from build123d import *

# Parameters (mm, degrees)
F0_W     = 88.9
F0_H     = 38.1
F1_DEPTH = 222.25
F2_R     = 9.525
F3_DEPTH = 12.7
F4_R     = 9.525
F5_DEPTH = 12.7


with BuildPart() as f1:
    # F0 (on Front) → F1 (new body, symmetric)
    with BuildSketch(Plane.XZ):
        Rectangle(F0_W, F0_H)
    extrude(amount=F1_DEPTH, both=True)

    # F2 (on face) → F3 (cut)
    with BuildSketch(Plane.XY.offset(19.05)):
        with Locations((0, 177.8)):
            Circle(F2_R)
        with Locations((0, -177.8)):
            Circle(F2_R)
    extrude(amount=-F3_DEPTH, mode=Mode.SUBTRACT)

    # F4 (on face) → F5 (cut)
    with BuildSketch(Plane(origin=(0, 0, -19.05), x_dir=(1, 0, 0), z_dir=(0, 0, -1))):
        with Locations((0, -177.8)):
            Circle(F4_R)
        with Locations((0, 177.8)):
            Circle(F4_R)
    extrude(amount=-F5_DEPTH, mode=Mode.SUBTRACT)


solid = f1.part
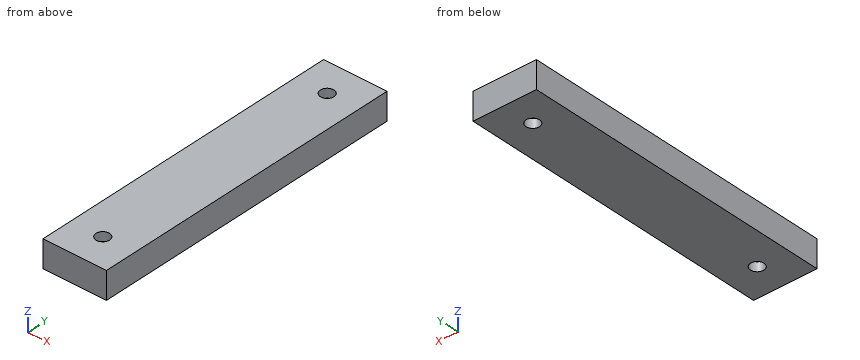
Here's how the part is built. I have some questions about the finished solid (model axes, mm). Coordinates: 2 decimals unless noted, no trailing zeros. Loops run counter-clockwise (first coordinate to the right, second up) from the corner with the lowest first, then second, coordinate; pieces in that order, holes last.
1. Imagine slicing it at A-A, the plane x = 0. Please give me the cut outline in (y, z) (3 decimals), and give its area (3 significant figures).
2. Imagine slicing it at B-B, the plane y = 177.8. Please give me the cut outline in (x, z) (3 decimals), and give its area (3 significant figures).
3. I need wall thicknesses on L1, parallel to Y at x = 0, z = -11 (3 decimals); L2, parallel to X at y = 177, z = 9. Which ranges of each line are inside material? Lowest first, please.
4. For P1, Ø17, axis at x = 0, y = 177.8, coming from the +Z side; P2, Ø17, axis at x = 0, y = -177.8, coming from the -Z side, each with a flat end and sliding along its axis, tell me the tip position at first contact or that it passes through.
Taken from the geometry:
1. outline: (-222.25, -19.05) - (-187.325, -19.05) - (-187.325, -6.35) - (-168.275, -6.35) - (-168.275, -19.05) - (168.275, -19.05) - (168.275, -6.35) - (187.325, -6.35) - (187.325, -19.05) - (222.25, -19.05) - (222.25, 19.05) - (187.325, 19.05) - (187.325, 6.35) - (168.275, 6.35) - (168.275, 19.05) - (-168.275, 19.05) - (-168.275, 6.35) - (-187.325, 6.35) - (-187.325, 19.05) - (-222.25, 19.05) - close
1. area: 16,000 mm2
2. outline: (-44.45, -19.05) - (-9.525, -19.05) - (-9.525, -6.35) - (9.525, -6.35) - (9.525, -19.05) - (44.45, -19.05) - (44.45, 19.05) - (9.525, 19.05) - (9.525, 6.35) - (-9.525, 6.35) - (-9.525, 19.05) - (-44.45, 19.05) - close
2. area: 2,900 mm2
3. L1: y = -222.25 to -187.325, -168.275 to 168.275, 187.325 to 222.25
3. L2: x = -44.45 to -9.49, 9.49 to 44.45
4. P1: stops at z = 6.35
4. P2: stops at z = -6.35
